from build123d import *

# Parameters (mm, degrees)
CROQUIS1_R              = 2.5
SALIENTE_EXTRUIR1_DEPTH = 10
REDONDEO1_RADIUS        = 2.5
REDONDEO1_LENGTH        = 10


with BuildPart() as part:
    # Croquis1 → Saliente-Extruir1 (new body)
    with BuildSketch(Plane(origin=(0, 0, 0), x_dir=(1, 0, 0), z_dir=(0, 1, 0))):
        with BuildLine():
            Line((-2.5, 8), (2.5, 8))
            Line((2.5, 8), (2.5, 3.122498999))
            ThreePointArc((2.5, 3.122498999), (0, -4), (-2.5, 3.122498999))
            Line((-2.5, 3.122498999), (-2.5, 8))
        make_face()
        with Locations(Location((0, 0, 0), (0, 0, 270))):
            Circle(CROQUIS1_R, mode=Mode.SUBTRACT)
    extrude(amount=SALIENTE_EXTRUIR1_DEPTH)

    # Redondeo1: full round fillet: the end face becomes a half cylinder, R = half its width
    redondeo1_face = Plane((0, 5, -8), x_dir=(0, 1, 0), z_dir=(0, 0, -1))  # on the end face: x along it, z out of the body
    redondeo1_slab = redondeo1_face.offset(-REDONDEO1_RADIUS / 2) * Box(REDONDEO1_LENGTH, 2 * REDONDEO1_RADIUS, REDONDEO1_RADIUS, mode=Mode.PRIVATE)  # the body's end, R deep
    redondeo1_round = Plane((0, 5, -5.5), x_dir=(0, 0, -1), z_dir=(0, 1, 0)) * Cylinder(REDONDEO1_RADIUS, REDONDEO1_LENGTH, mode=Mode.PRIVATE)  # its axis R under the face
    add(redondeo1_slab - redondeo1_round, mode=Mode.SUBTRACT)


solid = part.part
Model file for the job. Use its own axes, mm. A direction names the side the tool comes from. Give positions to 0.01 mm unless a question says otherwise; leave off trailing zeros. Order: outer loops, then holes, each group sorted by start corner. A loop starts at its lowest first (then second) coordinate and runs counter-clockwise, first axis right, second up. Notation, with made-up numbers: M 63,63 L 94,63 A25 ccw 94,92 Z; hole C -35.75,4 d9. An arc over 180 degrees is marked long. Put each result on its own line as item: value. Start each with the question number.
(1) Pull direction X, two halves, no side cores. Call faces 3 (the face through (0, 5, -8)), 4 (the face through (-2.5, 5, -4)), 5 (the face through (-2.44, 4.93, -0.54)): released by +X, released by -X, zero draft, split by the parting line, or undercut.
(2) Band-saw the part on B-B on z = 0. Give the cut face in (x, y), then the cut area to 3 significant figures.
(3) Drill centre lines: L1, parallel to X at y = 5.5, z = 0; L2, parallel to X at y = 1.75, z = -5.25; L3, parallel to Z at x = 0.75, y = 1.5. Where is each one in solid material? Low to high. Write a range as [from, to].
(4) Tool access for faces 1 (the face through (0, 5, 4)), 2 (the face through (2.5, 5, -4)): list every direction of +Z, -Z, +X, -X, +Y, -Y with a clear straight run to the whole face (end or side of a thin tool).
(5) Band-saw the part on D-D on z = 2.75. Give the cut face in (x, y).
(6) Band-saw the part on A-A on x = 0. Give the cut face in (y, z).
(7) Pin check, flat tips, straight feed: pin 1 Ø1.9 at (y, z) = (2.5, -4) entering from +X; pin 2 Ø1.9 at (y, z) = (2.5, -5) entering from -X. Stop position of each tip, or through.
(8) Band-saw the part on C-C on y = 5.25. Give the cut face in (x, z).
Results below:
1. face 3: split by the parting line
1. face 4: released by -X
1. face 5: undercut
2. outline: M -4,0 L -2.5,0 L -2.5,10 L -4,10 Z; M 2.5,0 L 4,0 L 4,10 L 2.5,10 Z
2. area: 30.0 mm2
3. L1: x = [-4, -2.5], [2.5, 4]
3. L2: x = [-2.5, 2.5]
3. L3: z = [-7.88, -2.38], [2.38, 3.93]
4. face 1: +Y, -Y
4. face 2: -Z, +X, +Y, -Y
5. outline: M -2.9,0 L 2.9,0 L 2.9,10 L -2.9,10 Z
6. outline: M 0,-8 L 10,-8 L 10,-2.5 L 0,-2.5 Z; M 0,2.5 L 10,2.5 L 10,4 L 0,4 Z
7. pin 1: stops at x = 2.59
7. pin 2: stops at x = -2.5
8. outline: M -2.5,-5.5 A2.5 ccw 2.5,-5.5 L 2.5,-3.12 A4 ccw long -2.5,-3.12 Z; hole C 0,0 d5
